```python
from build123d import *

# Parameters (mm, degrees)
PAD_DEPTH     = 2
SKETCH001_R   = 3.4
SKETCH001_W   = 7
SKETCH001_H   = 6.2
SKETCH001_W_2 = 6.2
SKETCH001_H_2 = 7
PAD001_DEPTH  = 7
CHAMFER_SIZE  = 1
FILLET_R      = 1


with BuildPart() as part:
    # Sketch → Pad (new body)
    with BuildSketch(Plane.XY):
        with BuildLine():
            Line((-13, 15), (13, 15))
            ThreePointArc((15, 13), (14.414214, 14.414214), (13, 15))
            Line((15, 13), (15, -13))
            ThreePointArc((13, -15), (14.414214, -14.414214), (15, -13))
            Line((13, -15), (-13, -15))
            ThreePointArc((-15, -13), (-14.414214, -14.414214), (-13, -15))
            Line((-15, -13), (-15, 13))
            ThreePointArc((-13, 15), (-14.414214, 14.414214), (-15, 13))
        make_face()
    extrude(amount=PAD_DEPTH)

    # Sketch001 → Pad001 (join)
    with BuildSketch(Plane.XY):
        Circle(SKETCH001_R)
        with Locations((-11.5, 0)):
            Rectangle(SKETCH001_W, SKETCH001_H)
        with Locations((0, -11.5)):
            Rectangle(SKETCH001_W_2, SKETCH001_H_2)
        with Locations((11.5, 0)):
            Rectangle(SKETCH001_W, SKETCH001_H)
        with Locations((0, 11.5)):
            Rectangle(SKETCH001_W_2, SKETCH001_H_2)
    extrude(amount=PAD001_DEPTH)

    # Chamfer
    chamfer_edges = [part.edges().sort_by_distance(p)[0] for p in [
        (-3.4, 0, 7),
        (-11.5, -3.1, 7),
        (-11.5, 3.1, 7),
        (-3.1, 11.5, 7),
        (3.1, 11.5, 7),
        (11.5, 3.1, 7),
        (11.5, -3.1, 7),
        (3.1, -11.5, 7),
        (-3.1, -11.5, 7),
    ]]
    chamfer(chamfer_edges, length=CHAMFER_SIZE)

    # Fillet
    fillet_edges = [part.edges().sort_by_distance(p)[0] for p in [
        (-3.4, 0, 2),
    ]]
    fillet(fillet_edges, radius=FILLET_R)


solid = part.part
```
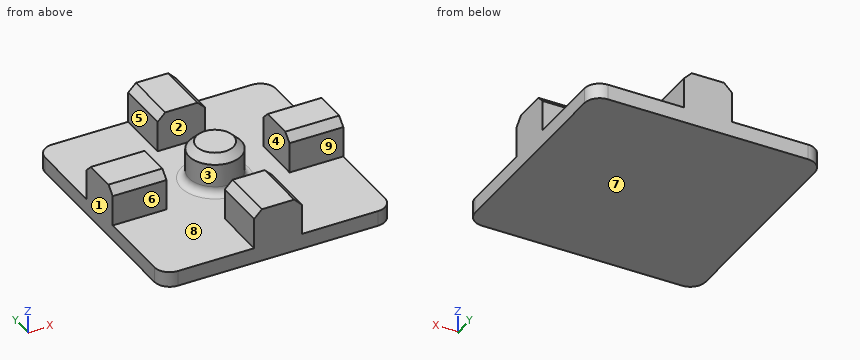
Source: CAD feature listing. Evaluate the final solid. Frame: model axes, mm. Face numbers are marked on the shaded views. A direction names the side the tool comes from. Give positions to 0.01 mm unless a question says otherwise; leave off trailing zeros. Loops run counter-clockwise (first coordinate to the right, second up) from the corner with the lowest first, then second, coordinate; pieces in that order, holes last. Notation, with made-up numbers: (64, 19.25) -> (113, 19.25) arc R29 ccw to (113, 48.25) -> close; hole circle Ø10 at (35, 11.25). An arc over 180 degrees is marked (long way). Use a Markdown table: item, result. Add a question column.
(1) Section query A-A (z = 4.25). Output: boundary loops of the cut face in (x, y).
(2) Section query B-B (x = 0). Output: boundary loops of the cut face in (y, z).
(3) First-contact query: pin 1 Ø5 at (x, y) = (9.5, -11.5) entering from -Z; pin 2 Ø3 at (y, z) = (-12, 4) entering from +X; pin 3 Ø2 at (x, z) = (-11, 5) entering from -Y; pin 4 Ø2 at (x, z) = (12, 4.5) entering from +Y. Flat tips, straight axial feed; report the tip coordinate or a pass-through.
(4) Access query for the marked faces 5, 6, 7, 8 and 9. Directions: +Z, -Z, +X, -X, +Y, -Y. A direction counts if a zero-diameter tool reaches every point of the face in a straight line with its end or side. Return the directions, or none.
(5) Pull-direction query (X, two-part tool) for the marked faces 1, 2, 3 and 4; classes: +X half, -X half, draft (parallel to the pull), parting line (faces both ways), or undercut.
(6) Ray query, line 1 (X direction, y = 3, z = 4.25); line 2 (Y direction, x = -1, z = 5.25); line 3 (Z direction, x = -12, y = 14.5). Return the intervals inside material, ascending.
(7) Section query C-C (y = -10.5). Output: boundary loops of the cut face in (x, z), then the cut area to 3 significant figures.
Checked values:
| question | item | result |
|---|---|---|
| 1 | outline | (-15, -3.1) -> (-8, -3.1) -> (-8, 3.1) -> (-15, 3.1) -> close; circle Ø6.8 at (0, 0); (-3.1, -15) -> (3.1, -15) -> (3.1, -8) -> (-3.1, -8) -> close; (-3.1, 8) -> (3.1, 8) -> (3.1, 15) -> (-3.1, 15) -> close; (8, -3.1) -> (15, -3.1) -> (15, 3.1) -> (8, 3.1) -> close |
| 2 | outline | (-15, 0) -> (15, 0) -> (15, 7) -> (8, 7) -> (8, 2) -> (4.4, 2) arc R1 cw to (3.4, 3) -> (3.4, 6) -> (2.4, 7) -> (-2.4, 7) -> (-3.4, 6) -> (-3.4, 3) arc R1 cw to (-4.4, 2) -> (-8, 2) -> (-8, 7) -> (-15, 7) -> close |
| 3 | pin 1 | z = 0 |
| 3 | pin 2 | x = 3.1 |
| 3 | pin 3 | y = -3.1 |
| 3 | pin 4 | y = 3.1 |
| 4 | face 5 | +Z, -X, +Y |
| 4 | face 6 | +Z, -X, -Y |
| 4 | face 7 | -Z, +X, -X, +Y, -Y |
| 4 | face 8 | +Z |
| 4 | face 9 | +Z, +X, -Y |
| 5 | face 1 | -X half |
| 5 | face 2 | draft |
| 5 | face 3 | undercut |
| 5 | face 4 | undercut |
| 6 | line 1 | -15 to -8, -1.6 to 1.6, 8 to 15 |
| 6 | line 2 | -15 to -8, -3.25 to 3.25, 8 to 15 |
| 6 | line 3 | 0 to 2 |
| 7 | outline | (-15, 0) -> (15, 0) -> (15, 2) -> (3.1, 2) -> (3.1, 6) -> (2.1, 7) -> (-2.1, 7) -> (-3.1, 6) -> (-3.1, 2) -> (-15, 2) -> close |
| 7 | area | 90.0 mm^2 |
